Here's how the part is built. I have some questions about the finished solid (model axes, mm). A direction names the side the tool comes from. Round coordinates to 2 decimals unless told otherwise and drop trailing zeros. Order: outer loops, then holes, each group sorted by start corner. A loop starts at its lowest first (then second) coordinate and runs counter-clockwise, first axis right, second up. Notation, with made-up numbers: (10.25, -25.5) -> (55.25, -25.5) arc R29 ccw to (55.25, -2.5) -> close; hole circle Ø9 at (-24.75, -21). An arc over 180 degrees is marked (long way). One line per item, written item: value.
```python
from build123d import *

# Parameters (mm, degrees)
SKETCH1_W           = 20
SKETCH1_H           = 40.5
BOSS_EXTRUDE1_DEPTH = 9.50000005
SKETCH2_W           = 20
SKETCH2_H           = 40.5
BOSS_EXTRUDE2_DEPTH = 17.1
SKETCH3_R           = 2.25
BOSS_EXTRUDE3_DEPTH = 2.5
SKETCH4_R           = 2.794
BOSS_EXTRUDE4_DEPTH = 6.702060002
SKETCH7_R           = 2.5
CUT_EXTRUDE1_DEPTH  = 2.54
BOSS_EXTRUDE6_DEPTH = 3.937


with BuildPart() as part:
    # Sketch1 → Boss-Extrude1 (new body, symmetric)
    with BuildSketch(Plane.XY):
        with Locations((10, 20.25)):
            Rectangle(SKETCH1_W, SKETCH1_H)
    extrude(amount=BOSS_EXTRUDE1_DEPTH, both=True)

    # Sketch2 → Boss-Extrude2 (add)
    with BuildSketch(Plane(origin=(0, 0, -9.50000005), x_dir=(-1, 0, 0), z_dir=(0, 0, -1))):
        with Locations((-10, 20.25)):
            Rectangle(SKETCH2_W, SKETCH2_H)
    extrude(amount=BOSS_EXTRUDE2_DEPTH)

    # Sketch3 → Boss-Extrude3 (add)
    with BuildSketch(Plane.XY):
        Polygon((19, 0), (19, -7.5), (1, -7.5), (1, 0), (0, 0), (0, 40.5), (1, 40.5), (1, 48), (19, 48), (19, 40.5), (20, 40.5), (20, 0), align=None)
        with Locations((5, -5)):
            Circle(SKETCH3_R, mode=Mode.SUBTRACT)
        with Locations((15, -5)):
            Circle(SKETCH3_R, mode=Mode.SUBTRACT)
        with Locations((5, 45.5)):
            Circle(SKETCH3_R, mode=Mode.SUBTRACT)
        with Locations((15, 45.5)):
            Circle(SKETCH3_R, mode=Mode.SUBTRACT)
    extrude(amount=BOSS_EXTRUDE3_DEPTH)

    # Sketch4 → Boss-Extrude4 (add)
    with BuildSketch(Plane.XY.offset(9.50000005)):
        with Locations((10, 30.1)):
            Circle(SKETCH4_R)
    extrude(amount=BOSS_EXTRUDE4_DEPTH)

    # Sketch7 → Cut-Extrude1 (cut)
    with BuildSketch(Plane(origin=(0, 40.5, 0), x_dir=(1, 0, 0), z_dir=(0, 1, 0))):
        with Locations((10, 17.60000005)):
            Circle(SKETCH7_R)
    extrude(amount=-CUT_EXTRUDE1_DEPTH, mode=Mode.SUBTRACT)

    # Sketch9 → Boss-Extrude6 (add)
    with BuildSketch(Plane(origin=(0, 0, -26.60000005), x_dir=(-1, 0, 0), z_dir=(0, 0, -1))):
        Polygon((-13.1115, 40.5), (-6.8885, 40.5), (-7.714, 46.342), (-12.286, 46.342), align=None)
    extrude(amount=-BOSS_EXTRUDE6_DEPTH)


solid = part.part
```
Q1. If we mould it in two halves opening along Y, with no side actions, what happens to faces 1 (the face through (17.146, -4.324, 1.232)), 2 (the face through (10, 30, 16.202)), 3 (the face through (12.693, 43.462, -24.659))? For each: pulls with the +Y half, pulls with the -Y half, needs draft (parallel to the pull), parting line crosses it, or undercut.
Answers:
face 1: undercut
face 2: needs draft
face 3: pulls with the +Y half
Q2. For P1, Ø4.5, axis at x = 10.5, z = -23.5, coming from the +Y side; P2, Ø1.2, axis at y = 44, z = 1.5, coming from the +X side; P3, Ø2.5, axis at x = 15, y = -5, coming from the -Z side; P4, Ø6.5, axis at x = 10, z = -17.6, coming from the -Y side, each with a flat end and sliding along its axis, tell me the tip position at first contact or that it passes through.
Answers:
P1: y = 46.34
P2: x = 19
P3: through
P4: y = 0
Q3. I want a section at A-A on y = -5. Write out the boundary of the cut face in (x, z).
Answers:
outline: (1, 0) -> (2.75, 0) -> (2.75, 2.5) -> (1, 2.5) -> close; (7.25, 0) -> (12.75, 0) -> (12.75, 2.5) -> (7.25, 2.5) -> close; (17.25, 0) -> (19, 0) -> (19, 2.5) -> (17.25, 2.5) -> close
Q4. I need wall thicknesses on line 1 along Y through (x, z) = (15, 1.05); line 2 along Z through (x, y) = (10, 39.6); line 3 along Y through (x, z) = (16.75, 1.5). Which ranges of each line are inside material? Lowest first, please.
Answers:
line 1: -7.5 to -7.25, -2.75 to 43.25, 47.75 to 48
line 2: -26.6 to -20.1, -15.1 to 9.5
line 3: -7.5 to -6.41, -3.59 to 44.09, 46.91 to 48
Q5. I want a section at C-C on z = -17.6. Write out the boundary of the cut face in (x, y), then the cut area to 3 significant figures.
Answers:
outline: (0, 0) -> (20, 0) -> (20, 40.5) -> (12.5, 40.5) -> (12.5, 37.96) -> (7.5, 37.96) -> (7.5, 40.5) -> (0, 40.5) -> close
area: 797 mm2
Q6. Which directions (+Z, -Z, +X, -X, +Y, -Y) give clear straight access to the entire face, cutting with the end or side of a thin tool? Please do faces 4 (the face through (9.46, 39.25, -15.16)), 5 (the face through (10, 43, -22.663)), 6 (the face through (1, -4, 1)), 7 (the face through (19, -4, 1)).
Answers:
face 4: +Y
face 5: +X, -X, +Y
face 6: +Z, -Z, -X, -Y
face 7: +Z, -Z, +X, -Y
Q7. I want a section at B-B on x = 14.75. Write out the boundary of the cut face in (y, z).
Answers:
outline: (-7.5, 0) -> (-7.24, 0) -> (-7.24, 2.5) -> (-7.5, 2.5) -> close; (-2.76, 0) -> (0, 0) -> (0, -26.6) -> (40.5, -26.6) -> (40.5, 0) -> (43.26, 0) -> (43.26, 2.5) -> (40.5, 2.5) -> (40.5, 9.5) -> (0, 9.5) -> (0, 2.5) -> (-2.76, 2.5) -> close; (47.74, 0) -> (48, 0) -> (48, 2.5) -> (47.74, 2.5) -> close
Q8. I want a section at D-D on y = 45.5. Write out the boundary of the cut face in (x, z).
Answers:
outline: (1, 0) -> (2.75, 0) -> (2.75, 2.5) -> (1, 2.5) -> close; (7.25, 0) -> (12.75, 0) -> (12.75, 2.5) -> (7.25, 2.5) -> close; (7.6, -26.6) -> (12.4, -26.6) -> (12.4, -22.66) -> (7.6, -22.66) -> close; (17.25, 0) -> (19, 0) -> (19, 2.5) -> (17.25, 2.5) -> close
